Geometry check sheet. Reference: the model listing, model coordinates, mm. A direction names the side the tool comes from. Give positions to 0.01 mm unless a question says otherwise; leave off trailing zeros. Loops run counter-clockwise (first coordinate to the right, second up) from the corner with the lowest first, then second, coordinate; pieces in that order, holes last. Notation, with made-up numbers: (2.5, 13) -> (42.5, 13) arc R28 cw to (42.5, 43) -> close; hole circle Ø8 at (64.5, 43). An arc over 180 degrees is marked (long way). Answer as a JSON object with one key per item and string values.
from build123d import *

# Parameters (mm, degrees)
BOSS_EXTRU_1_DEPTH              = 13
BOSS_EXTRU_1_DEPTH_BACK         = 12
COQUE1_T                        = -5
ESQUISSE3_R                     = 2.5
ENL_V_MAT_EXTRU_2_DEPTH         = 65
ESQUISSE5_R                     = 2.5
ENL_V_MAT_EXTRU_3_DEPTH         = 5
R_P_TITION_LIN_AIRE1_COUNT      = 2
R_P_TITION_LIN_AIRE1_PITCH      = 55
R_P_TITION_LIN_AIRE1_COUNT_DIR2 = 2
R_P_TITION_LIN_AIRE1_PITCH_DIR2 = 42
ENL_V_MAT_EXTRU_4_DEPTH         = 20
ESQUISSE8_W                     = 100
ESQUISSE8_H                     = 11.6
BOSS_EXTRU_2_DEPTH              = 5


with BuildPart() as part:
    # Esquisse1 → Boss.-Extru.1 (new body, two sides)
    with BuildSketch(Plane.XY) as boss_extru_1_sk:
        Polygon((44.118436308, 33.667601464), (51.949315251, 33.667601464), (51.949315251, -9.124565742), (29.741482457, -31.332398536), (-25.842851955, -31.332398536), (-48.050684749, -9.124565742), (-48.050684749, 33.667601464), align=None)
    extrude(amount=BOSS_EXTRU_1_DEPTH)
    extrude(boss_extru_1_sk.sketch, amount=-BOSS_EXTRU_1_DEPTH_BACK)

    # Coque1
    coque1_openings = [part.faces().sort_by_distance(p)[0] for p in [
        (1.949315251, -2.263120938, 13),
    ]]
    offset(amount=COQUE1_T, openings=coque1_openings, kind=Kind.INTERSECTION)

    # Esquisse3 → Enlèv. mat.-Extru.2 (cut)
    with BuildSketch(Plane.XZ.offset(31.332398536)):
        with Locations((-23.050684749, 8)):
            Circle(ESQUISSE3_R)
        with Locations((26.949315251, 8)):
            Circle(ESQUISSE3_R)
    extrude(amount=-ENL_V_MAT_EXTRU_2_DEPTH, mode=Mode.SUBTRACT)

    # Esquisse5 → Enlèv. mat.-Extru.3 (cut)
    with BuildSketch(Plane.XY.offset(-7)):
        with Locations((-25.550684749, 23.667601464)):
            Circle(ESQUISSE5_R)
    enl_v_mat_extru_3 = extrude(amount=-ENL_V_MAT_EXTRU_3_DEPTH, mode=Mode.SUBTRACT)

    # Répétition linéaire1: Enl_v. mat.-Extru.3 2 × 2
    with Locations(*[(i * R_P_TITION_LIN_AIRE1_PITCH, -j * R_P_TITION_LIN_AIRE1_PITCH_DIR2, 0) for i in range(R_P_TITION_LIN_AIRE1_COUNT) for j in range(R_P_TITION_LIN_AIRE1_COUNT_DIR2) if (i, j) != (0, 0)]):
        add(enl_v_mat_extru_3, mode=Mode.SUBTRACT)

    # Esquisse6 → Enlèv. mat.-Extru.4 (cut)
    with BuildSketch(Plane.XY.offset(13)):
        with BuildLine():
            Line((35.20468587, -18.798127311), (29.937348937, -24.065464245))
            ThreePointArc((29.937348937, -24.065464245), (34.372934866, -23.23371324), (35.20468587, -18.798127311))
        make_face()
        with BuildLine():
            Line((-31.365895508, -18.738287171), (-26.27917923, -23.825003449))
            ThreePointArc((-26.27917923, -23.825003449), (-30.493197573, -22.952305514), (-31.365895508, -18.738287171))
        make_face()
    extrude(amount=-ENL_V_MAT_EXTRU_4_DEPTH, mode=Mode.SUBTRACT)

    # Esquisse8 → Boss.-Extru.2 (add)
    with BuildSketch(Plane(origin=(0, 33.667601464, 0), x_dir=(1, 0, 0), z_dir=(0, 1, 0))):
        with Locations((1.949315251, 6.2)):
            Rectangle(ESQUISSE8_W, ESQUISSE8_H)
    extrude(amount=BOSS_EXTRU_2_DEPTH)


solid = part.part
1) Depth check by flat-ended pin: P1, Ø8, axis at x = 26.95, z = 8, coming from the +Y side; P2, Ø4.5, axis at x = 26.95, z = 8, coming from the +Y side; P3, Ø1.5, axis at x = 10, y = 35, coming from the +Z side; P4, Ø2, axis at x = 35, z = -6.5, coming from the -Y side. Enter the tip coordinate at first touch or a pass-through.
Geometry check:
{"P1": "stops at y = 33.67", "P2": "passes through", "P3": "stops at z = -0.4", "P4": "stops at y = -27.07"}
2) Section check A-A on z = 8. Count the separate pieces of the cut face and the enclosed holes in it, plus the area to 3 significant figures.
Geometry check:
{"separate pieces": "4", "enclosed holes": "0", "area": "1,300 mm2"}
3) Tool access check on faces 5 (the face through (2, 30, 13)), 6 (the face through (1, 36, -0.4)), 7 (the face through (2, -26.332, 3)). Record the directions out of +Z, -Z, +X, -X, +Y, -Y that give a thin tool (end or side, any length) a straight path to the whole face; none if there is none.
Geometry check:
{"face 5": "+Z, +X, -X, +Y, -Y", "face 6": "+Z, +X, -X, +Y", "face 7": "+Z"}
4) Material ranges on line 1 along X through (y, z) = (5.5, -0.5); line 2 along Y through (x, z) = (-14.5, 2.5); line 3 along Y through (x, z) = (18.5, -4.5), recorded low to high. Write a range as from..to.
Geometry check:
{"line 1": "x = -48.05..-43.05, 46.95..51.95", "line 2": "y = -31.33..-26.33, 28.67..33.67", "line 3": "y = -31.33..-26.33, 28.67..38.67"}
5) Section check D-D on x = 13. Record the cut outline in (y, z), plus the area to 3 significant figures.
Geometry check:
{"outline": "(-31.33, -12) -> (38.67, -12) -> (38.67, -0.4) -> (33.67, -0.4) -> (33.67, 13) -> (28.67, 13) -> (28.67, -7) -> (-26.33, -7) -> (-26.33, 13) -> (-31.33, 13) -> close", "area": "583 mm2"}
6) Section check B-B on z = -5.25. Record the cut outline in (x, y) (1 decimal).
Geometry check:
{"outline": "(-48.1, -9.1) -> (-25.8, -31.3) -> (29.7, -31.3) -> (51.9, -9.1) -> (51.9, 38.7) -> (-48.1, 38.7) -> close; hole (-43.1, -7.1) -> (-31.4, -18.7) arc R3.9 ccw to (-26.3, -23.8) -> (-23.8, -26.3) -> (27.7, -26.3) -> (29.9, -24.1) arc R4 ccw to (35.2, -18.8) -> (46.9, -7.1) -> (46.9, 28.7) -> (-43.1, 28.7) -> close"}
7) Draft check along X on faces 1 (the face through (2, -31.332, 1)), 2 (the face through (46.949, 11, 3)), 3 (the face through (-23.59, 31.13, 5.56)), 4 (the face through (-48.051, 14, 1)). Enter one of: pulls with the +X half, pulls with the -X half, needs draft (parallel to the pull), parting line crosses it, or undercut.
Geometry check:
{"face 1": "needs draft", "face 2": "undercut", "face 3": "undercut", "face 4": "pulls with the -X half"}
8) Section check C-C on y = 8. Record the cut outline in (x, z), plus the area to 3 significant figures.
Geometry check:
{"outline": "(-48.05, -12) -> (51.95, -12) -> (51.95, 13) -> (46.95, 13) -> (46.95, -7) -> (-43.05, -7) -> (-43.05, 13) -> (-48.05, 13) -> close", "area": "700 mm2"}
